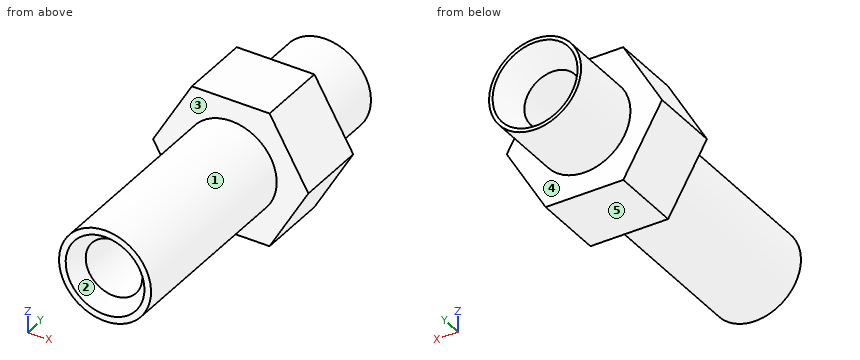
from build123d import *

# Parameters (mm, degrees)
BOSS_EXTRUDE1_DEPTH      = 10
BOSS_EXTRUDE2_DEPTH      = 11
BOSS_EXTRUDE2_DEPTH_BACK = 38
SKETCH2_R                = 6.5
SKETCH3_R                = 4
CUT_EXTRUDE1_DEPTH       = 57
CHAMFER1_SIZE            = 2
CHAMFER1_SIZE2           = 3.925221011
CHAMFER2_SIZE            = 2
CHAMFER2_SIZE2           = 1.562571253


with BuildPart() as part:
    # Sketch1 → Boss-Extrude1 (new body)
    with BuildSketch(Plane(origin=(0, 0, 0), x_dir=(1, 0, 0), z_dir=(0, 1, 0))):
        Polygon((10.969655115, 0), (5.484827557, 9.5), (-5.484827557, 9.5), (-10.969655115, 0), (-5.484827557, -9.5), (5.484827557, -9.5), align=None)
    extrude(amount=BOSS_EXTRUDE1_DEPTH)

    # Sketch2 → Boss-Extrude2 (add, two sides: drawn at the far end of the back side and taken through both)
    with BuildSketch(Plane(origin=(0, 10, 0), x_dir=(1, 0, 0), z_dir=(0, 1, 0)).offset(-BOSS_EXTRUDE2_DEPTH_BACK)):
        with Locations(Location((0, 0, 0), (0, 0, 270))):
            Circle(SKETCH2_R)
    extrude(amount=BOSS_EXTRUDE2_DEPTH + BOSS_EXTRUDE2_DEPTH_BACK)

    # Sketch3 → Cut-Extrude1 (cut)
    with BuildSketch(Plane(origin=(0, 21, 0), x_dir=(1, 0, 0), z_dir=(0, 1, 0))):
        with Locations(Location((0, 0, 0), (0, 0, 270))):
            Circle(SKETCH3_R)
    extrude(amount=-CUT_EXTRUDE1_DEPTH, mode=Mode.SUBTRACT)

    # Chamfer1
    chamfer1_edges = [part.edges().sort_by_distance(p)[0] for p in [
        (0, 21, -4),
    ]]
    chamfer1_side = [part.faces().sort_by_distance(p)[0] for p in [
        (0, 21, -6.316152237),
    ]]
    chamfer(chamfer1_edges, length=CHAMFER1_SIZE, length2=CHAMFER1_SIZE2, reference=chamfer1_side[0])

    # Chamfer2
    chamfer2_edges = [part.edges().sort_by_distance(p)[0] for p in [
        (0, -28, -4),
    ]]
    chamfer2_side = [part.faces().sort_by_distance(p)[0] for p in [
        (0, -5.462610506, -4),
    ]]
    chamfer(chamfer2_edges, length=CHAMFER2_SIZE, length2=CHAMFER2_SIZE2, reference=chamfer2_side[0])


solid = part.part
The model under review builds one solid part; all positions refer to its coordinate system, in mm. Face numbers are marked on the shaded views. A direction names the side the tool comes from. Round coordinates to 2 decimals unless told otherwise and drop trailing zeros. Loops run counter-clockwise (first coordinate to the right, second up) from the corner with the lowest first, then second, coordinate; pieces in that order, holes last. Notation, with made-up numbers: (45, 28) -> (99, 28) arc R21 cw to (99, 60) -> close; hole circle Ø11 at (83, -38.5). An arc over 180 degrees is marked (long way). Return JSON: item names as keys, results as strings.
(1) Add section B-B on y = -20. Write out the cut boundary in (x, z), plus the area to 3 significant figures.
Solved:
{"outline": "circle Ø13 at (0, 0); hole circle Ø8 at (0, 0)", "area": "82.5 mm2"}
(2) For the marked faces 4 and 5, list the 3-axis set-ups (+Z, -Z, +X, -X, +Y, -Y) from which the entire face can be reached by the end or side of a thin tool; tool diameter is ignored.
Solved:
{"face 4": "+Y", "face 5": "-Z, +X, -X, +Y, -Y"}
(3) Add section A-A on x = 0. Write out the cut boundary in (y, z).
Solved:
{"outline": "(-28, -6.5) -> (0, -6.5) -> (0, -9.5) -> (10, -9.5) -> (10, -6.5) -> (21, -6.5) -> (21, -6) -> (17.07, -4) -> (-26, -4) -> (-28, -5.56) -> close; (-28, 5.56) -> (-26, 4) -> (17.07, 4) -> (21, 6) -> (21, 6.5) -> (10, 6.5) -> (10, 9.5) -> (0, 9.5) -> (0, 6.5) -> (-28, 6.5) -> close"}
(4) For line 1 (X direction, y = 6.5, z = 0); line 2 (X direction, y = -3, z = 0); line 3 (Y direction, x = -3.5, z = -7), list the stretches that pass through material, from the lowest coordinate up.
Solved:
{"line 1": "-10.97 to -4, 4 to 10.97", "line 2": "-6.5 to -4, 4 to 6.5", "line 3": "0 to 10"}
(5) The part is to be moulded in two halves that separate along Z. For the marked faces 1, 2 and 3, say which applies: released by +Z, released by -Z, zero draft, split by the parting line, or undercut.
Solved:
{"face 1": "split by the parting line", "face 2": "undercut", "face 3": "zero draft"}
(6) Add section C-C on x = -9.5. Write out the cut boundary in (y, z), plus the area to 3 significant figures.
Solved:
{"outline": "(0, -2.55) -> (10, -2.55) -> (10, 2.55) -> (0, 2.55) -> close", "area": "50.9 mm2"}
(7) For pin 1 (1 mm diameter, centred on y = -17.5, z = -5, fed in from +X); pin 2 (2 mm diameter, centred on y = -14.5, z = 0.5, fed in from -X); pin 3 (1.5 mm diameter, centred on x = 4.5, z = 6.5, fed in from +Y), all flat-tipped, find the tip position at first contact; note any pin that passes through.
Solved:
{"pin 1": "x = 4.69", "pin 2": "x = -6.5", "pin 3": "y = 10"}
